Read the model definition and answer for the solid it produces. Units are mm, in the model's axes. Face numbers are marked on the shaded views. Round coordinates to 2 decimals unless told otherwise and drop trailing zeros. Loops run counter-clockwise (first coordinate to the right, second up) from the corner with the lowest first, then second, coordinate; pieces in that order, holes last. Notation, with made-up numbers: (83.5, -19.75) - (109.5, -19.75) arc R18 ccw to (109.5, -7.75) - close; hole circle Ø1 at (2.5, 51). An arc over 180 degrees is marked (long way). Use one line per item in the form item = value. Start each with the question number.
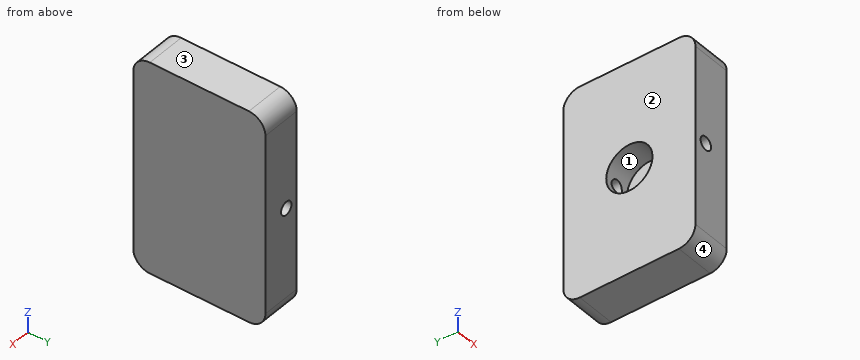
```python
from build123d import *

# Parameters (mm, degrees)
EXTRUDE_1_DEPTH     = 12
SKETCH_2_R          = 7
CUT_EXTRUDE_1_DEPTH = 8
SKETCH_5_R          = 2
CUT_EXTRUDE_2_DEPTH = 41


with BuildPart() as part:
    # 草图1 → 凸台-拉伸1 (new body)
    with BuildSketch(Plane(origin=(0, 0, 0), x_dir=(0, 0, -1), z_dir=(1, 0, 0))):
        with BuildLine():
            Line((-27, 20), (27, 20))
            ThreePointArc((27, 20), (30.535533906, 18.535533906), (32, 15))
            Line((32, 15), (32, -15))
            ThreePointArc((32, -15), (30.535533906, -18.535533906), (27, -20))
            Line((27, -20), (-27, -20))
            ThreePointArc((-27, -20), (-30.535533906, -18.535533906), (-32, -15))
            Line((-32, -15), (-32, 15))
            ThreePointArc((-32, 15), (-30.535533906, 18.535533906), (-27, 20))
        make_face()
    extrude(amount=EXTRUDE_1_DEPTH)

    # 草图2 → 切除-拉伸1 (cut)
    with BuildSketch(Plane.ZY):
        Circle(SKETCH_2_R)
    extrude(amount=-CUT_EXTRUDE_1_DEPTH, mode=Mode.SUBTRACT)

    # 草图5 → 切除-拉伸2 (cut, through all)
    with BuildSketch(Plane.XZ.offset(20)):
        with Locations((4, 0)):
            Circle(SKETCH_5_R)
    extrude(amount=-CUT_EXTRUDE_2_DEPTH, mode=Mode.SUBTRACT)


solid = part.part
```
1) A cutting plane is placed at A-A on x = 4. Write down the section's boundary in (y, z).
2) A cutting plane is placed at D-D on y = 0. Write down the section's boundary in (x, z), plus the area to 3 significant figures.
3) Straight lines are drawn through the part: line 1 (Z direction, x = 4, y = 10.5); line 2 (X direction, y = 15.25, z = 0); line 3 (Y direction, x = 2.75, z = -4). For each, find the intervals that lie inside material, in ascending order. Write a range as from..to.
4) A cutting plane is placed at C-C on z = 0. Write down the section's boundary in (x, y).
5) Determine the mould class of the marked faces 1, 2, 3 and 4 for opening direction Z: +Z half, -Z half, draft (parallel to the pull), parting line (faces both ways), or undercut.
6) A cutting plane is placed at B-B on x = 1.25. Write down the section's boundary in (y, z).
Checks:
q1.outline = (-20, -27) arc R5 ccw to (-15, -32) - (15, -32) arc R5 ccw to (20, -27) - (20, -2) - (6.71, -2) arc R7 cw to (-6.71, -2) - (-20, -2) - close; (-20, 2) - (-6.71, 2) arc R7 cw to (6.71, 2) - (20, 2) - (20, 27) arc R5 ccw to (15, 32) - (-15, 32) arc R5 ccw to (-20, 27) - close
q2.outline = (0, -32) - (12, -32) - (12, 32) - (0, 32) - (0, 7) - (8, 7) - (8, -7) - (0, -7) - close
q2.area = 656 mm²
q3.line_1 = -32..-2, 2..32
q3.line_2 = 0..2, 6..12
q3.line_3 = -20..-5.74, 5.74..20
q4.outline = (0, -20) - (2, -20) - (2, -7) - (0, -7) - close; (0, 7) - (2, 7) - (2, 20) - (0, 20) - close; (6, -20) - (12, -20) - (12, 20) - (6, 20) - (6, 7) - (8, 7) - (8, -7) - (6, -7) - close
q5.face_1 = undercut
q5.face_2 = draft
q5.face_3 = +Z half
q5.face_4 = -Z half
q6.outline = (-20, -27) arc R5 ccw to (-15, -32) - (15, -32) arc R5 ccw to (20, -27) - (20, 27) arc R5 ccw to (15, 32) - (-15, 32) arc R5 ccw to (-20, 27) - close; hole circle Ø14 at (0, 0)
